Autodesk Inventor part; units mm, degrees
ref_plane "YZ Plane" through (0, 0, 0) normal (1, 0, 0) x (0, 1, 0)
ref_plane "XZ Plane" through (0, 0, 0) normal (0, 1, 0) x (-1, 0, 0)
ref_plane "XY Plane" through (0, 0, 0) normal (0, 0, 1) x (1, 0, 0)
sketch "Sketch1" plane through (0, 0, 0) normal (0, 0, 1) x (1, 0, 0)
  line L0 (0, 0) -> (160, 0)
  line L1 (160, 0) -> (160, 50)
  line L2 (160, 50) -> (0, 50)
  line L3 (0, 50) -> (0, 0)
  line L4 (50, 0) -> (110, 0)
  line L5 (110, 0) -> (110, 8.3313)
  line L6 (110, 8.3313) -> (50, 8.3313)
  line L7 (50, 8.3313) -> (50, 0)
  line L8 (0, 50) -> (160, 50)
  line L9 (160, 50) -> (160, 45)
  line L10 (0, 45) -> (0, 50)
  line L11 (150, 50) -> (10, 50)
  line L12 (10, 30) -> (150, 30)
  line L13 (150, 30) -> (150, 25)
  line L14 (150, 25) -> (10, 25)
  line L15 (10, 25) -> (10, 30)
  dimension "d0" = 160
  dimension "d1" = 50
  dimension "d2" = 60
  dimension "d3" = 50
  dimension "d11" = 140
  dimension "d12" = 10
  dimension "d13" = 20
  dimension "d14" = 5
extrude "Extrusion1" add sketch "Sketch1" along normal blind 5 contours L3 L2 L1 L0 L5 L6 L7 | L12 L13 L14 L15
extrude "Extrusion2" add sketch "Sketch1" against normal blind 65 contours L12 L13 L14 L15
sketch "Sketch2" plane through (0, 0, 5) normal (0, 0, 1) x (1, 0, 0)
  line L0 (160, 50) -> (0, 50)
  line L1 (70, 50) -> (85, 50)
  line L2 (85, 50) -> (85, 70)
  line L3 (85, 70) -> (70, 70)
  line L4 (70, 70) -> (70, 50)
  line L5 (72, 68) -> (83, 68)
  line L6 (83, 68) -> (83, 52)
  line L7 (83, 52) -> (72, 52)
  line L8 (72, 52) -> (72, 68)
  point P0 (0, 0)
  dimension "d15" = 15
  dimension "d16" = 20
  dimension "d17" = 2
extrude "Extrusion3" add sketch "Sketch2" against normal blind 5
sketch "Sketch3" plane through (0, 0, 5) normal (0, 0, 1) x (1, 0, 0)
  point P0 (0, 0)
properties part number "COVER_1" material "ABS Plastic"
Here's how the part is built. I have some questions about the finished solid (model axes, mm). A direction names the side the tool comes from. Give positions to 0.01 mm unless a question says otherwise; leave off trailing zeros. Loops run counter-clockwise (first coordinate to the right, second up) from the corner with the lowest first, then second, coordinate; pieces in that order, holes last. Notation, with made-up numbers: M 59.25,-6.5 L 100.25,-6.5 A24 cw 100.25,22.5 Z; hole C -12,12 d6. An arc over 180 degrees is marked long. Put each result on its own line as item: value. Start each with the question number.
(1) I want a section at B-B on y = 58. Please give me the cut outline in (x, z), then the cut area to 3 significant figures.
(2) For faces 5 (the flat face through (10, 27, -32)), 6 (the flat face through (70, 60, 3)), 7 (the flat face through (78, 52, 3)), 8 (the flat face through (80, 8.331, 2)), 9 (the flat face through (79, 30, -32)), which set-ups out of +Z, -Z, +X, -X, +Y, -Y let a thin tool reach every point of the face, with its end or its side?
(3) I want a section at A-A on x = 65. Please give me the cut outline in (y, z).
(4) If we mould it in two halves opening along Y, with no side actions, what happens to faces 1 (the flat face through (81, 25, -32)), 2 (the flat face through (78, 70, 3)), 3 (the flat face through (160, 25, 2)), 4 (the flat face through (72, 60, 3))? For each: +Y half, -Y half, draft (parallel to the pull), parting line (faces both ways), or undercut.
(5) I want a section at C-C on y = 42.5. Please give me the cut outline in (x, z).
(6) I want a section at D-D on z = -11. Please give me the cut outline in (x, y).
(7) I need wall thicknesses on line 1 along Z through (x, y) = (130.5, 34.5); line 2 along Y through (x, z) = (76, -60). Which ranges of each line are inside material? Lowest first, please. Write a range as [from, to].
(8) Will these pins go through, and if not, where does the flat tip stop? pin 1 Ø12 at (x, z) = (53.5, -45) entering from -Y; pin 2 Ø21 at (x, y) = (48, 51.5) entering from -Z; pin 3 Ø2.5 at (y, z) = (56.5, 1.5) entering from -X.
Answer block:
1. outline: M 70,0 L 72,0 L 72,5 L 70,5 Z; M 83,0 L 85,0 L 85,5 L 83,5 Z
1. area: 20.0 mm^2
2. face 5: -Z, -X, +Y, -Y
2. face 6: +Z, -Z, -X, +Y
2. face 7: +Z, -Z
2. face 8: +Z, -Z, -Y
2. face 9: -Z, +X, -X, +Y
3. outline: M 8.33,0 L 25,0 L 25,-65 L 30,-65 L 30,0 L 50,0 L 50,5 L 8.33,5 Z
4. face 1: -Y half
4. face 2: +Y half
4. face 3: draft
4. face 4: undercut
5. outline: M 0,0 L 160,0 L 160,5 L 0,5 Z
6. outline: M 10,25 L 150,25 L 150,30 L 10,30 Z
7. line 1: [0, 5]
7. line 2: [25, 30]
8. pin 1: y = 25
8. pin 2: z = 0
8. pin 3: x = 70
